Autodesk Inventor part; units mm, degrees
ref_plane "YZ Plane" through (0, 0, 0) normal (1, 0, 0) x (0, 1, 0)
ref_plane "XZ Plane" through (0, 0, 0) normal (0, 1, 0) x (-1, 0, 0)
ref_plane "XY Plane" through (0, 0, 0) normal (0, 0, 1) x (1, 0, 0)
sketch "Sketch1" plane through (0, 0, 0) normal (0, 0, 1) x (1, 0, 0)
  line L0 (-26.62, 18.8707) -> (74.98, 18.8707)
  line L1 (74.98, 18.8707) -> (74.98, 12.5207)
  line L2 (74.98, -83.9993) -> (-26.62, -83.9993)
  line L3 (-26.62, -83.9993) -> (-26.62, 18.8707)
  line L4 (-26.62, 18.8707) -> (24.18, 18.8707)
  line L5 (24.18, 18.8707) -> (24.18, -33.1993)
  line L6 (24.18, -33.1993) -> (1.32, -33.1993)
  line L7 (24.18, -33.1993) -> (67.36, -33.1993)
  line L8 (1.32, -33.1993) -> (1.32, 12.5207)
  line L9 (1.32, 12.5207) -> (67.36, 12.5207)
  line L10 (67.36, 12.5207) -> (67.36, -33.1993)
  circle A0 centre (24.18, -33.1993) radius 12.7
  line L11 (74.98, 18.8707) -> (82.6, 18.8707)
  line L12 (82.6, 18.8707) -> (82.6, -83.9993)
  line L13 (82.6, -83.9993) -> (74.98, -83.9993)
  line L14 (1.32, -33.1993) -> (1.32, -77.6493)
  line L15 (1.32, 12.5207) -> (-5.03, 12.5207)
  line L16 (-5.03, 12.5207) -> (-5.03, -12.8793)
  line L17 (-5.03, -12.8793) -> (1.32, -12.8793)
  line L18 (1.32, -77.6493) -> (-5.03, -77.6493)
  line L19 (-5.03, -77.6493) -> (-5.03, -52.2493)
  line L20 (-5.03, -52.2493) -> (1.32, -52.2493)
  line L21 (1.32, -77.6493) -> (1.32, -45.2643)
  line L22 (1.32, -45.2643) -> (-5.03, -45.2643)
  line L23 (-5.03, -45.2643) -> (-5.03, -19.8643)
  line L24 (-5.03, -19.8643) -> (1.32, -19.8643)
  line L25 (67.36, -33.1993) -> (67.36, -77.6493)
  line L26 (67.36, -77.6493) -> (73.71, -77.6493)
  line L27 (73.71, -77.6493) -> (73.71, -52.2493)
  line L28 (73.71, -52.2493) -> (67.36, -52.2493)
  line L29 (67.36, -52.2493) -> (67.36, -45.2643)
  line L30 (67.36, -45.2643) -> (73.71, -45.2643)
  line L31 (73.71, -45.2643) -> (73.71, -19.8643)
  line L32 (73.71, -19.8643) -> (67.36, -19.8643)
  line L33 (67.36, 12.5207) -> (73.71, 12.5207)
  line L34 (73.71, 12.5207) -> (73.71, -12.8793)
  line L35 (73.71, -12.8793) -> (67.36, -12.8793)
  point P0 (0, 0)
  dimension "d0" = 101.6
  dimension "d1" = 102.87
  dimension "d2" = 50.8
  dimension "d3" = 52.07
  dimension "d4" = 22.86
  dimension "d5" = 43.18
  dimension "d6" = 45.72
  dimension "d7" = 25.4
  dimension "d8" = 7.62
  dimension "d9" = 44.45
  dimension "d10" = 6.35
  dimension "d11" = 25.4
  dimension "d12" = 6.35
  dimension "d13" = 25.4
  dimension "d14" = 32.385
  dimension "d15" = 25.4
  dimension "d16" = 6.35
  dimension "d17" = 25.4
  dimension "d18" = 6.985
  dimension "d19" = 25.4
extrude "Extrusion1" add sketch "Sketch1" along normal blind 6.35 contours L9 L10 L7 A0 L5 | L5 A0 L6 L8 L9 | L0 L11 L12 L13 L2 L3 | A0 L7 L5 | L5 L6 A0 | L7 A0 L6
sketch "Sketch2" plane through (0, 0, 6.35) normal (0, 0, 1) x (1, 0, 0)
  arc A0 (11.48, -33.1993) -> (36.88, -33.1993) centre (24.18, -33.1993) ccw
  line L0 (36.88, -33.1993) -> (11.48, -33.1993)
  circle A1 centre (24.18, -33.1993) radius 12.7
  point P0 (0, 0)
  dimension "d22" = 25.4
extrude "Extrusion2" cut sketch "Sketch2" against normal blind 6.35 contours A1 L0
sketch "Sketch3" plane through (0, 0, 6.35) normal (0, 0, 1) x (1, 0, 0)
  line L0 (-26.62, 18.8707) -> (82.6, 18.8707)
  line L1 (82.6, -83.9993) -> (-26.62, -83.9993)
  line L2 (-26.62, 18.8707) -> (-20.6637, 18.8707)
  line L3 (-20.6637, 18.8707) -> (-20.6637, 12.9144)
  line L4 (-26.62, -83.9993) -> (-20.6637, -83.9993)
  line L5 (-20.6637, -83.9993) -> (-20.6637, -78.043)
  line L6 (-26.62, 18.8707) -> (74.98, 18.8707)
  circle A0 centre (-20.6637, 12.9144) radius 1.9812
  circle A1 centre (-20.6637, -78.043) radius 1.9812
  point P0 (0, 0)
  dimension "d25" = 5.9563
  dimension "d26" = 5.9563
  dimension "d27" = 5.9563
  dimension "d28" = 5.9563
  dimension "d29" = 101.6
  dimension "d30" = 3.9624
  dimension "d31" = 3.9624
extrude "Extrusion3" cut sketch "Sketch3" against normal blind 6.35
sketch "Sketch4" plane through (0, 0, 6.35) normal (0, 0, 1) x (1, 0, 0)
  line L0 (67.36, 12.5207) -> (73.71, 12.5207)
  line L1 (73.71, 12.5207) -> (73.71, -12.8793)
  line L2 (67.36, -12.8793) -> (67.36, 12.5207)
  line L3 (1.32, 12.5207) -> (1.32, -12.8793)
  line L4 (-5.03, -12.8793) -> (-5.03, 12.5207)
  line L5 (-5.03, 12.5207) -> (1.32, 12.5207)
  line L6 (-5.03, 12.5207) -> (-5.03, -0.1793)
  line L7 (-5.03, -0.1793) -> (1.32, -0.1793)
  line L8 (67.36, 12.5207) -> (67.36, -0.1793)
  line L9 (67.36, -0.1793) -> (73.71, -0.1793)
  point P0 (0, 0)
  dimension "d34" = 12.7
  dimension "d35" = 12.7
extrude "Extrusion4" add sketch "Sketch4" against normal blind 6.35
sketch "Sketch5" plane through (0, 0, 6.35) normal (0, 0, 1) x (1, 0, 0)
  circle A0 centre (-20.6637, 12.9144) radius 1.9812
  line L0 (-26.62, 18.8707) -> (82.6, 18.8707)
  line L1 (82.6, -83.9993) -> (-26.62, -83.9993)
  line L2 (73.71, -52.2493) -> (73.71, -77.6493)
  line L3 (67.36, -77.6493) -> (67.36, -52.2493)
  line L4 (67.36, -0.1793) -> (73.71, -0.1793)
  line L5 (-5.03, -0.1793) -> (1.32, -0.1793)
  line L6 (-26.62, 18.8707) -> (74.98, 18.8707)
  line L7 (74.98, 18.8707) -> (74.98, 12.9144)
  line L8 (-26.62, -83.9993) -> (74.98, -83.9993)
  line L9 (-5.03, -0.1793) -> (-5.03, 12.5207)
  line L10 (-5.03, 12.5207) -> (1.32, 12.5207)
  line L11 (1.32, 12.5207) -> (1.32, -0.1793)
  line L12 (67.36, -77.6493) -> (67.36, -70.0293)
  line L13 (67.36, -70.0293) -> (73.71, -70.0293)
  line L14 (67.36, -0.1793) -> (67.36, 4.9007)
  line L15 (67.36, 4.9007) -> (73.71, 4.9007)
  line L16 (73.71, 4.9007) -> (73.71, -0.1793)
  point P0 (0, 0)
  dimension "d38" = 101.6
  dimension "d39" = 5.9563
  dimension "d40" = 5.9563
  dimension "d41" = 101.6
  dimension "d42" = 12.7
  dimension "d43" = 7.62
  dimension "d44" = 5.08
extrude "Extrusion5" cut sketch "Sketch5" against normal blind 6.35 contours L14 L15 L16 L4 | L9 L10 L11 L5
sketch "Sketch6" plane through (0, 0, 6.35) normal (0, 0, 1) x (1, 0, 0)
  line L0 (73.71, -52.2493) -> (73.71, -77.6493)
  line L1 (73.71, -77.6493) -> (67.36, -77.6493)
  line L2 (67.36, -77.6493) -> (67.36, -52.2493)
  line L3 (67.36, -77.6493) -> (67.36, -70.0293)
  line L4 (67.36, -70.0293) -> (73.71, -70.0293)
  point P0 (0, 0)
  dimension "d47" = 7.62
extrude "Extrusion6" add sketch "Sketch6" against normal blind 6.35
sketch "Sketch7" plane through (0, 0, 6.35) normal (0, 0, 1) x (1, 0, 0)
  line L0 (-26.62, 18.8707) -> (82.6, 18.8707)
  line L1 (82.6, -83.9993) -> (-26.62, -83.9993)
  line L2 (-26.62, 18.8707) -> (74.98, 18.8707)
  line L3 (74.98, 18.8707) -> (74.98, 12.9144)
  line L4 (-26.62, -83.9993) -> (74.98, -83.9993)
  line L5 (74.98, -83.9993) -> (74.98, -78.043)
  line L6 (74.98, -78.043) -> (69.0237, -78.043)
  line L7 (74.98, 12.9144) -> (69.0237, 12.9144)
  circle A0 centre (69.0237, 12.9144) radius 1.9812
  circle A1 centre (69.0237, -78.043) radius 1.9812
  point P0 (0, 0)
  dimension "d50" = 101.6
  dimension "d51" = 5.9563
  dimension "d52" = 101.6
  dimension "d53" = 5.9563
  dimension "d54" = 5.9563
  dimension "d55" = 5.9563
  dimension "d56" = 3.9624
  dimension "d57" = 3.9624
extrude "Extrusion7" cut sketch "Sketch7" against normal blind 6.35
sketch "Sketch8" plane through (0, 0, 6.35) normal (0, 0, 1) x (1, 0, 0)
  line L0 (73.71, 4.9007) -> (73.71, -12.8793)
  line L1 (-26.62, 18.8707) -> (82.6, 18.8707)
  line L2 (82.6, -83.9993) -> (-26.62, -83.9993)
  line L3 (82.6, 18.8707) -> (82.6, -83.9993)
  line L4 (73.71, -52.2493) -> (73.71, -70.0293)
  line L5 (73.71, -19.8643) -> (73.71, -45.2643)
  line L6 (-26.62, 18.8707) -> (74.98, 18.8707)
  line L7 (74.98, 18.8707) -> (74.98, -83.9993)
  line L8 (73.71, -52.2493) -> (74.98, -52.2493)
  line L9 (73.71, -70.0293) -> (74.98, -70.0293)
  line L10 (73.71, -45.2643) -> (74.98, -45.2643)
  line L11 (73.71, -19.8643) -> (74.98, -19.8643)
  line L12 (73.71, 4.9007) -> (74.98, 4.9007)
  line L13 (73.71, -12.8793) -> (74.98, -12.8793)
  point P0 (0, 0)
  dimension "d60" = 101.6
extrude "Extrusion8" cut sketch "Sketch8" against normal blind 6.35
sketch "Sketch9" plane through (0, 0, 6.35) normal (0, 0, 1) x (1, 0, 0)
  line L0 (74.98, -45.2643) -> (67.36, -45.2643)
  line L1 (67.36, -45.2643) -> (67.36, -19.8643)
  line L2 (67.36, -19.8643) -> (74.98, -19.8643)
  line L3 (-5.03, 12.5207) -> (1.32, 12.5207)
  line L4 (74.98, -19.8643) -> (74.98, -45.2643)
  point P0 (0, 0)
extrude "Extrusion9" add sketch "Sketch9" against normal blind 6.35
sketch "Sketch11" plane through (0, 0, 6.35) normal (0, 0, 1) x (1, 0, 0)
  line L0 (67.36, 4.9007) -> (74.98, 4.9007)
  line L1 (74.98, -83.9993) -> (74.98, -70.0293)
  line L2 (67.36, -70.0293) -> (67.36, -52.2493)
  line L3 (74.98, -52.2493) -> (74.98, -12.8793)
  line L4 (67.36, -12.8793) -> (67.36, 4.9007)
  line L5 (-5.03, 12.5207) -> (1.32, 12.5207)
  line L6 (67.36, 4.9007) -> (67.36, -20.4993)
  line L7 (67.36, -20.4993) -> (74.98, -20.4993)
  line L8 (74.98, 4.9007) -> (74.98, -20.4993)
  line L9 (74.98, 4.9007) -> (67.36, 4.9007)
  line L10 (67.36, -70.0293) -> (67.36, -44.6293)
  line L11 (67.36, -44.6293) -> (74.98, -44.6293)
  line L12 (74.98, -44.6293) -> (74.98, -70.0293)
  line L13 (67.36, -70.0293) -> (74.98, -70.0293)
  point P0 (0, 0)
  dimension "d67" = 25.4
  dimension "d68" = 25.4
  dimension "d69" = 7.62
extrude "Extrusion10" cut sketch "Sketch11" against normal blind 6.35
sketch "Sketch12" plane through (0, 0, 6.35) normal (0, 0, 1) x (1, 0, 0)
  line L0 (1.32, -19.8643) -> (1.32, -45.2643)
  line L1 (1.32, -45.2643) -> (-5.03, -45.2643)
  line L2 (-5.03, -45.2643) -> (-5.03, -19.8643)
  line L3 (-5.03, -19.8643) -> (1.32, -19.8643)
  point P0 (0, 0)
extrude "Extrusion11" add sketch "Sketch12" against normal blind 6.35
sketch "Sketch13" plane through (0, 0, 6.35) normal (0, 0, 1) x (1, 0, 0)
  circle A0 centre (24.18, -33.1993) radius 12.7
  point P0 (0, 0)
extrude "Extrusion12" add sketch "Sketch13" against normal blind 6.35
sketch "Sketch14" plane through (0, 0, 6.35) normal (0, 0, 1) x (1, 0, 0)
  circle A0 centre (69.0237, -78.043) radius 1.9812
  circle A1 centre (69.0237, 12.9144) radius 1.9812
  circle A2 centre (-20.6637, -78.043) radius 1.9812
  circle A3 centre (-20.6637, 12.9144) radius 1.9812
  point P0 (0, 0)
extrude "Extrusion13" add sketch "Sketch14" against normal blind 6.35
sketch "Sketch15" plane through (0, 0, 6.35) normal (0, 0, 1) x (1, 0, 0)
  line L0 (74.98, 4.9007) -> (74.98, 18.8707)
  line L1 (74.98, -83.9993) -> (74.98, -70.0293)
  line L2 (-26.62, 18.8707) -> (74.98, 18.8707)
  line L3 (74.98, 18.8707) -> (74.98, 18.2357)
  line L4 (74.98, 18.2357) -> (-26.62, 18.2357)
  line L5 (-26.62, 18.2357) -> (-26.62, 18.8707)
  line L6 (-26.62, -83.9993) -> (74.98, -83.9993)
  line L7 (74.98, -83.9993) -> (74.98, -83.3643)
  line L8 (74.98, -83.3643) -> (-26.62, -83.3643)
  line L9 (-26.62, -83.3643) -> (-26.62, -83.9993)
  point P0 (0, 0)
  dimension "d78" = 0.635
  dimension "d79" = 0.635
extrude "Extrusion14" cut sketch "Sketch15" against normal blind 6.35
sketch "Sketch16" plane through (0, 0, 6.35) normal (0, 0, 1) x (1, 0, 0)
  line L0 (-26.62, -83.3643) -> (-26.62, 18.2357)
  line L1 (-26.62, 18.2357) -> (74.98, -83.3643)
  line L2 (-26.62, -83.3643) -> (74.98, 18.2357)
  line L3 (-26.62, 18.2357) -> (-26.62, -32.5643)
  line L4 (-26.62, -32.5643) -> (-26.62, 12.2794)
  line L5 (-26.62, 12.2794) -> (69.0237, 12.2794)
  line L6 (69.0237, 12.2794) -> (69.0237, -77.408)
  line L7 (69.0237, -77.408) -> (-20.6637, -77.408)
  circle A0 centre (-20.6637, 12.2794) radius 1.9812
  circle A1 centre (69.0237, 12.2794) radius 1.9812
  circle A2 centre (69.0237, -77.408) radius 1.9812
  circle A3 centre (-20.6637, -77.408) radius 1.9812
  point P0 (0, 0)
  dimension "d82" = 50.8
  dimension "d83" = 44.8437
  dimension "d84" = 3.9624
  dimension "d85" = 3.9624
  dimension "d86" = 3.9624
  dimension "d87" = 3.9624
extrude "Extrusion15" cut sketch "Sketch16" against normal blind 6.35 contours A3 L2 | L2 L7 A3 | L2 A3 L7 | A0 L1 L5 | L5 L1 A0 | A2 L1 L7 | L7 L1 A2 | A0 L5 L1 | L5 A0 L1 | A2 L6 L1 | A1 L5 L2 | L2 L6 A1 | L6 A2 L1 | L5 A1 L2 | L2 A1 L6
sketch "Sketch17" plane through (0, 0, 0) normal (0, 0, -1) x (-1, 0, 0)
  line L0 (26.62, -83.3643) -> (-74.98, 18.2357)
  line L1 (26.62, 18.2357) -> (-74.98, -83.3643)
  circle A0 centre (-24.18, -32.5643) radius 12.7
  point P0 (0, 0)
  dimension "d90" = 25.4
extrude "Extrusion16" cut sketch "Sketch17" against normal blind 25.4
properties part number "wheel top"
Model file for the job. Use its own axes, mm. A direction names the side the tool comes from. Give positions to 0.01 mm unless a question says otherwise; leave off trailing zeros. Loops run counter-clockwise (first coordinate to the right, second up) from the corner with the lowest first, then second, coordinate; pieces in that order, holes last. Notation, with made-up numbers: (-33, 28) - (10, 28) arc R33 ccw to (10, 57) - close; hole circle Ø10 at (11.25, 18.25). An arc over 180 degrees is marked (long way). One line per item, written item: value. Start each with the question number.
1. Pin check, flat tips, straight feed: pin 1 (15 mm diameter, centred on x = 24.18, y = -32.56, fed in from +Z); pin 2 (3 mm diameter, centred on y = -10, z = 2, fed in from +X); pin 3 (5 mm diameter, centred on x = -20.66, y = 12.28, fed in from -Z). Stop position of each tip, or through.
2. Slice it at C-C (z = 2.5). List the corners of the cut face in (x, y), plus the area to 3 significant figures.
3. Pull direction X, two halves, no side cores. Call faces 4 (the flat face through (25, -83.364, 3)), 5 (the flat face through (74.98, 12, 3)), 6 (the flat face through (1.32, -65, 3)): pulls with the +X half, pulls with the -X half, needs draft (parallel to the pull), parting line crosses it, or undercut.
4. Slice it at B-B (x = 24.18). List the corners of the cut face in (y, z).
5. Probe L1, parallel to Y at x = -3.5, z = 4; L2, parallel to X at y = 0, z = 4.25; L3, parallel to X at y = -32, z = 0.5. List the from-to ranges inside material, lowest first. Write a range as from..to.
6. Slice it at A-A (y = -4.5). List the corners of the cut face in (x, z).
7. Which spindle directions (+Z, -Z, +X, -X, +Y, -Y) get a long thin tool onto all of the face, cutting with end or side? Do faces 1 (the flat face through (12, -21, 0)), 2 (the flat face through (-5.03, -65, 3)), 3 (the flat face through (71, -20.499, 3)). Say none if no direction does.
Solution:
1. pin 1: passes through
1. pin 2: stops at x = 67.36
1. pin 3: stops at z = 0
2. outline: (-26.62, -83.36) - (74.98, -83.36) - (74.98, -70.03) - (67.36, -70.03) - (67.36, -44.63) - (74.98, -44.63) - (74.98, -20.5) - (67.36, -20.5) - (67.36, 4.9) - (74.98, 4.9) - (74.98, 18.24) - (-26.62, 18.24) - close; hole circle Ø3.96 at (-20.66, -77.41); hole circle Ø3.96 at (-20.66, 12.28); hole (-5.03, -77.65) - (1.32, -77.65) - (1.32, -52.25) - (-5.03, -52.25) - close; hole (-5.03, -12.88) - (1.32, -12.88) - (1.32, 12.52) - (-5.03, 12.52) - close; hole circle Ø25.4 at (24.18, -32.56); hole circle Ø3.96 at (69.02, -77.41); hole circle Ø3.96 at (69.02, 12.28)
2. area: 9,060 mm^2
3. face 4: needs draft
3. face 5: pulls with the +X half
3. face 6: undercut
4. outline: (-83.36, 0) - (-45.26, 0) - (-45.26, 6.35) - (-83.36, 6.35) - close; (-19.86, 0) - (18.24, 0) - (18.24, 6.35) - (-19.86, 6.35) - close
5. L1: y = -83.36..-77.65, -52.25..-12.88, 12.52..18.24
5. L2: x = -26.62..-5.03, 1.32..67.36
5. L3: x = -26.62..11.49, 36.87..74.98
6. outline: (-26.62, 0) - (-5.03, 0) - (-5.03, 6.35) - (-26.62, 6.35) - close; (1.32, 0) - (67.36, 0) - (67.36, 6.35) - (1.32, 6.35) - close
7. face 1: -Z, +X, -X, +Y, -Y
7. face 2: +Z, -Z
7. face 3: +Z, -Z, +X
